```python
from build123d import *

# Parameters (mm, degrees)
ESQUISSE1_R        = 60
ESQUISSE1_W        = 250
ESQUISSE1_H        = 65
BOSS_EXTRU_1_DEPTH = 10


with BuildPart() as part:
    # Esquisse1 → Boss.-Extru.1 (new body)
    with BuildSketch(Plane.XY):
        Circle(ESQUISSE1_R)
        Rectangle(ESQUISSE1_W, ESQUISSE1_H)
    extrude(amount=BOSS_EXTRU_1_DEPTH)


solid = part.part
```
Can you work these out from the model? Positions are in its coordinate system, mm. A direction names the side the tool comes from. Give positions to 0.01 mm unless a question says otherwise; leave off trailing zeros. Order: outer loops, then holes, each group sorted by start corner. A loop starts at its lowest first (then second) coordinate and runs counter-clockwise, first axis right, second up. Notation, with made-up numbers: (-25.5, 5.25) - (-21.5, 5.25) arc R19 ccw to (-21.5, 32.25) - close; hole circle Ø11 at (-21.75, 83.5). An arc over 180 degrees is marked (long way). Use a Markdown table: item, result. Add a question column.
Q1. If we section it at C-C on y = 39: Write out the boundary of the cut face in (x, z), plus the area to 3 significant figures.
Q2. I'm going to push flat-ended pins straight in: pin 1 (5 mm diameter, centred on x = -96, z = 4, fed in from +Y); pin 2 (2 mm diameter, centred on y = 47.5, z = 2, fed in from +X); pin 3 (3 mm diameter, centred on x = -88.5, z = 4, fed in from -Y). Where does each tip first touch, or does it pass through?
Q3. If we section it at A-A on z = 1.5: Write out the boundary of the cut face in (x, y).
Q4. On a 3-axis mill with a long thin cutter (end or side, diameter ignored), from which of +Z, -Z, +X, -X, +Y, -Y can I reach the whole of each face in a straight line? I mean faces 1 (the flat face through (-88, 32.5, 5)), 2 (the flat face through (87, -32.5, 5)), 3 (the flat face through (87, 32.5, 5)). Say none if no direction works.
Q5. Please list where these lines run through material, in increasing order: line 1 along Y through (x, z) = (-84.5, 7.25); line 2 along X through (y, z) = (-49.5, 9.25); line 3 along Y through (x, z) = (-15, 8).
Q6. If we section it at B-B on x = 98.5: Write out the boundary of the cut face in (y, z), plus the area to 3 significant figures.
Answers follow:
| question | item | result |
|---|---|---|
| 1 | outline | (-45.6, 0) - (45.6, 0) - (45.6, 10) - (-45.6, 10) - close |
| 1 | area | 912 mm^2 |
| 2 | pin 1 | stops at y = 32.5 |
| 2 | pin 2 | stops at x = 37.92 |
| 2 | pin 3 | stops at y = -32.5 |
| 3 | outline | (-125, -32.5) - (-50.44, -32.5) arc R60 ccw to (50.44, -32.5) - (125, -32.5) - (125, 32.5) - (50.44, 32.5) arc R60 ccw to (-50.44, 32.5) - (-125, 32.5) - close |
| 4 | face 1 | +Z, -Z, -X, +Y |
| 4 | face 2 | +Z, -Z, +X, -Y |
| 4 | face 3 | +Z, -Z, +X, +Y |
| 5 | line 1 | y = -32.5 to 32.5 |
| 5 | line 2 | x = -33.91 to 33.91 |
| 5 | line 3 | y = -58.09 to 58.09 |
| 6 | outline | (-32.5, 0) - (32.5, 0) - (32.5, 10) - (-32.5, 10) - close |
| 6 | area | 650 mm^2 |
